```python
from build123d import *

# Parameters (mm, degrees)
EXTRUDE_THIN1_DEPTH = 192.5
CUT_EXTRUDE1_DEPTH  = 410.266930903
BOSS_EXTRUDE1_REACH = 238.446
SKETCH3_R           = 6.35


with BuildPart() as part:
    # Sketch1 → Extrude-Thin1 (new, symmetric)
    with BuildSketch(Plane(origin=(0, 0, 0), x_dir=(0, 0, -1), z_dir=(1, 0, 0))):
        with BuildLine():
            ThreePointArc((43.474740585, -93.231882052), (86.759678031, -55.272010711), (102.87, 0))
            Line((102.87, 0), (100.33, 0))
            ThreePointArc((100.33, 0), (84.617463758, -53.907269705), (42.4012902, -90.929860273))
            Line((42.4012902, -90.929860273), (43.474740585, -93.231882052))
        make_face()
    extrude(amount=EXTRUDE_THIN1_DEPTH, both=True)

    # Sketch2 → Cut-Extrude1 (cut, through all)
    with BuildSketch(Plane(origin=(192.5, 0, 0), x_dir=(0, 0, -1), z_dir=(1, 0, 0))):
        with BuildLine():
            Line((42.4012902, -90.929860273), (48.104026969, -90.929860273))
            ThreePointArc((48.104026969, -90.929860273), (45.803848013, -92.109958241), (43.474740585, -93.231882052))
            Line((43.474740585, -93.231882052), (42.4012902, -90.929860273))
        make_face()
    extrude(amount=-CUT_EXTRUDE1_DEPTH, mode=Mode.SUBTRACT)

    # Sketch3 → Boss-Extrude1 (add, up to next)
    with BuildSketch(Plane.XZ.offset(90.929860273), mode=Mode.PRIVATE) as boss_extrude1_sk1:
        with Locations(Location((-129, -96.52, 0), (0, 0, 270))):
            Circle(SKETCH3_R)
    boss_extrude1_tool1 = extrude(boss_extrude1_sk1.sketch, amount=-BOSS_EXTRUDE1_REACH, mode=Mode.PRIVATE) - part.part
    # Sketch3 → Boss-Extrude1 (add, up to next)
    with BuildSketch(Plane.XZ.offset(90.929860273), mode=Mode.PRIVATE) as boss_extrude1_sk2:
        with Locations(Location((129, -96.52, 0), (0, 0, 270))):
            Circle(SKETCH3_R)
    boss_extrude1_tool2 = extrude(boss_extrude1_sk2.sketch, amount=-BOSS_EXTRUDE1_REACH, mode=Mode.PRIVATE) - part.part
    # Sketch3 → Boss-Extrude1 (add, up to next)
    with BuildSketch(Plane.XZ.offset(90.929860273), mode=Mode.PRIVATE) as boss_extrude1_sk3:
        with Locations(Location((0, -96.52, 0), (0, 0, 270))):
            Circle(SKETCH3_R)
    boss_extrude1_tool3 = extrude(boss_extrude1_sk3.sketch, amount=-BOSS_EXTRUDE1_REACH, mode=Mode.PRIVATE) - part.part
    add(boss_extrude1_tool1.solids().sort_by_distance((-129, -90.92986, -96.52))[0])
    add(boss_extrude1_tool2.solids().sort_by_distance((129, -90.92986, -96.52))[0])
    add(boss_extrude1_tool3.solids().sort_by_distance((0, -90.92986, -96.52))[0])


solid = part.part
```
Model file for the job. Use its own axes, mm. A direction names the side the tool comes from. Give positions to 0.01 mm unless a question says otherwise; leave off trailing zeros. Write each loop counter-clockwise with the first axis right and the second up, starting at its lowest first coordinate (ties: lowest second). Pieces come first, ordered by that corner, then holes. Notation, with made-up numbers: (-30.75, 12.5) -> (-9.75, 12.5) arc R9 cw to (-9.75, 21.5) -> close; hole circle Ø9 at (33.5, 2). An arc over 180 degrees is marked (long way). Use CSV: the item, a comma, the result in double quotes. Start each with the question number.
1) Cut at C-C on y = -25.5. List the corners of the cut face in (x, z).
2) Cut at D-D on z = -96.52. List the corners of the cut face in (x, y), plus the area to 3 significant figures.
3) Cut at B-B on x = -11. List the corners of the cut face in (y, z), plus the area to 3 significant figures.
4) Pin check, flat tips, straight feed: P1, Ø8, axis at x = 72.5, y = -46.5, coming from the -Z side; P2, Ø6, axis at x = 118.5, z = -79, coming from the -Y side; P3, Ø5, axis at x = 62, z = -62.5, coming from the -Y side. Stop position of each tip, or through.
5) Drill centre lines: L1, parallel to Y at x = -116.5, z = -81; L2, parallel to Z at x = -100.5, y = -47; L3, parallel to Z at x = -89, y = -7. Where is each one in solid material? Low to high.
6) Two-plate mould, pull along Z, no slides. Class faces 1 (the cylindrical face through (130.907, -56.205, -102.577)), 2 (the cylindrical face through (2.695, -53.234, -85.043)), 3 (the cylindrical face through (-127.093, -56.205, -102.577)), 4 (the flat face through (-192.5, -52, -86)): released by +Z, released by -Z, zero draft, split by the parting line, or undercut.
7) Cut at A-A on y = -65. List the corners of the cut face in (x, z).
8) Tool access for faces 5 (the flat face through (0, -90.93, -96)), 6 (the cylindrical face through (2.695, -53.742, -87.716)): list every direction of +Z, -Z, +X, -X, +Y, -Y with a clear straight run to the whole face (end or side of a thin tool).
Final values:
1,outline,"(-192.5, -99.66) -> (-134.52, -99.66) arc R6.35 ccw to (-123.48, -99.66) -> (-5.52, -99.66) arc R6.35 ccw to (5.52, -99.66) -> (123.48, -99.66) arc R6.35 ccw to (134.52, -99.66) -> (192.5, -99.66) -> (192.5, -97.04) -> (-192.5, -97.04) -> close"
2,outline,"(-192.5, -35.58) -> (-135.35, -35.58) -> (-135.35, -90.93) -> (-122.65, -90.93) -> (-122.65, -35.58) -> (-6.35, -35.58) -> (-6.35, -90.93) -> (6.35, -90.93) -> (6.35, -35.58) -> (122.65, -35.58) -> (122.65, -90.93) -> (135.35, -90.93) -> (135.35, -35.58) -> (192.5, -35.58) -> (192.5, -27.39) -> (-192.5, -27.39) -> close"
2,area,"5,260 mm2"
3,outline,"(-90.93, -48.1) arc R102.87 ccw to (0, -102.87) -> (0, -100.33) arc R100.33 cw to (-90.93, -42.4) -> close"
3,area,"286 mm2"
4,P1,"stops at z = -93.68"
4,P2,"stops at y = -69.33"
4,P3,"stops at y = -83.56"
5,L1,"y = -63.41 to -59.2"
5,L2,"z = -91.51 to -88.64"
5,L3,"z = -102.63 to -100.09"
6,face 1,"undercut"
6,face 2,"released by +Z"
6,face 3,"undercut"
6,face 4,"zero draft"
7,outline,"(-192.5, -79.73) -> (192.5, -79.73) -> (192.5, -76.43) -> (-192.5, -76.43) -> close; circle Ø12.7 at (-129, -96.52); circle Ø12.7 at (0, -96.52); circle Ø12.7 at (129, -96.52)"
8,face 5,"+Z, -Z, +X, -X, -Y"
8,face 6,"-Y"
